```python
from build123d import *

# Parameters (mm, degrees)
F0_W          = 18
F0_H          = 32
F1_DEPTH      = 14
F2_W          = 13
F2_H          = 5
F2_W_2        = 2
F2_H_2        = 18.5
F3_DEPTH      = 14
F4_W          = 27
F4_H          = 6.5
F5_DEPTH      = 18.001
F6_R          = 1
F7_DEPTH      = 7.5
F8_R          = 1.25
F9_DEPTH      = 5
F10_T4_DEPTH  = 5
F11_T4_DEPTH  = 8.1066017178
F11_T9_DEPTH  = 8.1066017178
F11_T12_DEPTH = 20
F11_T14_DEPTH = 11.2132034356
F12_R         = 1
F13_T1_DEPTH  = 42.1410161514
F13_T3_DEPTH  = 42.5
F15_DEPTH     = 14.001
F16_R         = 1


# Not quite as in the source:
# - a fillet or chamfer that OpenCascade refuses, or shapes differently, is made with other operations: its cross-section is extruded or revolved along the edge and cut away or added


with BuildPart() as f1:
    # F0 (on Top) → F1 (new body)
    with BuildSketch(Plane.XY):
        with Locations((9, 16)):
            Rectangle(F0_W, F0_H)
    extrude(amount=F1_DEPTH)

    # F2 (on face) → F3 (cut, through all)
    with BuildSketch(Plane.XY.offset(14)):
        with Locations((11.5, 2.5)):
            Rectangle(F2_W, F2_H)
        with Locations((1, 22.75)):
            Rectangle(F2_W_2, F2_H_2)
    extrude(amount=-F3_DEPTH, mode=Mode.SUBTRACT)

    # F4 (on face) → F5 (cut, through all)
    with BuildSketch(Plane.YZ.offset(18)):
        with Locations((18.5, 3.25)):
            Rectangle(F4_W, F4_H)
    extrude(amount=-F5_DEPTH, mode=Mode.SUBTRACT)

    # F6 (on face) → F7 (cut, through all)
    with BuildSketch(Plane.XY.offset(14)):
        with Locations((13.5, 9.5)):
            Circle(F6_R)
        with BuildLine():
            ThreePointArc((18, 23.1904157598), (15.9251079936, 24.5306592691), (13.5, 25))
            ThreePointArc((13.5, 25), (7, 18.5), (13.5, 12))
            ThreePointArc((13.5, 12), (15.9251079936, 12.4693407309), (18, 13.8095842402))
            Line((18, 13.8095842402), (18, 23.1904157598))
        make_face()
        with Locations((13.5, 27.5)):
            Circle(F6_R)
        with BuildLine():
            Line((18, 25), (13.5, 25))
            ThreePointArc((13.5, 25), (15.9251079936, 24.5306592691), (18, 23.1904157598))
            Line((18, 23.1904157598), (18, 25))
        make_face()
        with BuildLine():
            ThreePointArc((18, 13.8095842402), (15.9251079936, 12.4693407309), (13.5, 12))
            Line((13.5, 12), (18, 12))
            Line((18, 12), (18, 13.8095842402))
        make_face()
    extrude(amount=-F7_DEPTH, mode=Mode.SUBTRACT)

    # F8 (on face) → F9 (cut, through all)
    with BuildSketch(Plane.YZ.offset(5)):
        with Locations((2.5, 11.55)):
            Circle(F8_R)
        with Locations((2.5, 2.95)):
            Circle(F8_R)
    extrude(amount=-F9_DEPTH, mode=Mode.SUBTRACT)

    # F10: chamfer of 8 on 1 edges, made by hand


with BuildPart() as f10_tool2:
    # F10_s3 → F10_t4 (new body)
    with BuildSketch(Plane.YZ.offset(5)):
        Polygon((5, -1.5), (13, 6.5), (5, 6.5), align=None)
    extrude(amount=-F10_T4_DEPTH)

    split(bisect_by=Plane.XY, keep=Keep.TOP)


with BuildPart() as f1_1:
    add(f1.part)

    # F10_t1: union F10_tool2
    add(f10_tool2.part)

    # F11: fillet of radius 3 on 5 edges, made by hand


with BuildPart() as f11_tool2:
    # F11_s3 → F11_t4 (new body)
    with BuildSketch(Plane.YZ.offset(5)):
        with BuildLine():
            ThreePointArc((14.2426406871, 6.5), (13.09459039, 6.2716385975), (12.1213203436, 5.6213203436))
            Line((12.1213203436, 5.6213203436), (13, 6.5))
            Line((13, 6.5), (14.2426406871, 6.5))
        make_face()
    extrude(amount=-F11_T4_DEPTH)

    split(bisect_by=Plane.YZ.offset(2), keep=Keep.TOP)


with BuildPart() as f1_2:
    add(f1_1.part)

    # F11_t1: union F11_tool2
    add(f11_tool2.part)


with BuildPart() as f11_tool7:
    # F11_s8 → F11_t9 (new body)
    with BuildSketch(Plane.YZ.offset(8.1066017178)):
        with BuildLine():
            ThreePointArc((14.2426406871, 6.5), (13.09459039, 6.2716385975), (12.1213203436, 5.6213203436))
            Line((12.1213203436, 5.6213203436), (13, 6.5))
            Line((13, 6.5), (14.2426406871, 6.5))
        make_face()
    extrude(amount=-F11_T9_DEPTH)

    split(bisect_by=Plane.YZ.offset(2), keep=Keep.BOTTOM)

    split(bisect_by=Plane.XZ.offset(-13.5), keep=Keep.TOP)


with BuildPart() as f1_3:
    add(f1_2.part)

    # F11_t6: union F11_tool7
    add(f11_tool7.part)

    # F11_s13 → F11_t12 (cut)
    with BuildSketch(Plane.YZ.offset(-7.5)):
        with BuildLine():
            ThreePointArc((0, 11), (0.8786796564, 13.1213203436), (3, 14))
            Line((3, 14), (0, 14))
            Line((0, 14), (0, 11))
        make_face()
        with BuildLine():
            ThreePointArc((0, 3), (0.8786796564, 0.8786796564), (3, 0))
            Line((3, 0), (0, 0))
            Line((0, 0), (0, 3))
        make_face()
    extrude(amount=F11_T12_DEPTH, mode=Mode.SUBTRACT)

    # F11_s15 → F11_t14 (cut)
    with BuildSketch(Plane.YZ.offset(-3.1066017178)):
        with BuildLine():
            ThreePointArc((7.3786796564, 0.8786796564), (6.40540961, 0.2283614025), (5.2573593129, 0))
            Line((5.2573593129, 0), (6.5, 0))
            Line((6.5, 0), (7.3786796564, 0.8786796564))
        make_face()
    extrude(amount=F11_T14_DEPTH, mode=Mode.SUBTRACT)

    # F12
    f12_edges = [f1_3.edges().sort_by_distance(p)[0] for p in [
        (18, 12, 10.25),
        (18, 25, 10.25),
    ]]
    fillet(f12_edges, radius=F12_R)

    # F13: fillet of radius 7 on 3 edges, made by hand

    # F13_s2 → F13_t1 (cut)
    with BuildSketch(Plane.XY.offset(-10.8205080757)):
        with BuildLine():
            ThreePointArc((18, 11), (15.6543724647, 6.7084973779), (11.0717967697, 5))
            Line((11.0717967697, 5), (11.0717967697, 4.86))
            Line((11.0717967697, 4.86), (18, 4.86))
            Line((18, 4.86), (18.14, 5))
            ThreePointArc((18.14, 5), (18.14, 8), (18.1385640646, 10.98))
            Line((18.1385640646, 10.98), (18, 11))
        make_face()
        with BuildLine():
            ThreePointArc((18, 26), (15.6543724647, 30.2915026221), (11.0717967697, 32))
            Line((11.0717967697, 32), (11.0717967697, 32.14))
            Line((11.0717967697, 32.14), (18, 32.14))
            Line((18, 32.14), (18.14, 32))
            ThreePointArc((18.14, 32), (18.14, 29), (18.1385640646, 26.02))
            Line((18.1385640646, 26.02), (18, 26))
        make_face()
    extrude(amount=F13_T1_DEPTH, mode=Mode.SUBTRACT)

    # F13_s4 → F13_t3 (cut)
    with BuildSketch(Plane.XY.offset(-11)):
        with BuildLine():
            ThreePointArc((9, 32), (4.0502525317, 29.9497474683), (2, 25))
            Line((2, 25), (1.86, 25))
            Line((1.86, 25), (1.86, 32.14))
            Line((1.86, 32.14), (9, 32.14))
            Line((9, 32.14), (9, 32))
        make_face()
    extrude(amount=F13_T3_DEPTH, mode=Mode.SUBTRACT)

    # F14 (on face) → F15 (cut, through all)
    with BuildSketch(Plane.XY.offset(14)):
        with BuildLine():
            ThreePointArc((8.1908098546, 14.75), (7, 18.5), (8.1908098546, 22.25))
            Line((8.1908098546, 22.25), (5.9908098546, 22.25))
            Line((5.9908098546, 22.25), (5.9908098546, 14.75))
            Line((5.9908098546, 14.75), (8.1908098546, 14.75))
        make_face()
    extrude(amount=-F15_DEPTH, mode=Mode.SUBTRACT)

    # F16
    f16_edges = [f1_3.edges().sort_by_distance(p)[0] for p in [
        (5.99081, 14.75, 10.25),
        (5.99081, 22.25, 10.25),
        (8.19081, 22.25, 10.25),
        (8.19081, 14.75, 10.25),
        (0, 13.5, 10.203314),
    ]]
    fillet(f16_edges, radius=F16_R)


solid = f1_3.part
```
Source: CAD feature listing. Evaluate the final solid. Frame: model axes, mm. A direction names the side the tool comes from. Give positions to 0.01 mm unless a question says otherwise; leave off trailing zeros. Write each loop counter-clockwise with the first axis right and the second up, starting at its lowest first coordinate (ties: lowest second). Pieces come first, ordered by that corner, then holes.
1. Section query C-C (x = 14). Return the cut outline in (y, z).
2. Section query B-B (y = 27.5). Return the cut outline in (x, z), then the cut area to 3 significant figures.
3. Section query D-D (x = 11.75). Return the cut outline in (y, z).
4. Pull-direction query (Y, two-part tool) for faces 1 (the face through (2.535, 3.077, 1.841)), 2 (the face through (5, 18, 14)), 3 (the face through (8, 5, 10)), 4 (the face through (10.681, 12.643, 10.302)); classes: +Y half, -Y half, draft (parallel to the pull), parting line (faces both ways), or undercut.
5. First-contact query: pin 1 (1.8 mm diameter, centred on x = 15.5, z = 9.5, fed in from -Y); pin 2 (5 mm diameter, centred on x = 9, z = 10.5, fed in from -Y); pin 3 (6 mm diameter, centred on y = 19.5, z = 11, fed in from -X). Flat tips, straight axial feed; report the tip coordinate or a pass-through.
6. Section query A-A (z = 11.55). Count the separate pieces of the cut face and the enclosed holes in it, then the cut area to 3 significant figures.
7. Material intervals for line 1 along Y through (x, z) = (13.5, 10.5); line 2 along Z through (x, y) = (3.7, 2.5); line 3 along X through (y, z) = (21, 8.5), sorted ascending.
8. Access query for faces 5 (the face through (17.715, 25.301, 10.198)), 6 (the face through (5, 18, 6.5)), 7 (the face through (3.091, 12.872, 6.169)), 8 (the face through (2, 19, 10)). Directions: +Z, -Z, +X, -X, +Y, -Y. A direction counts if a zero-diameter tool reaches every point of the face in a straight line with its end or side. Return the directions, or none.
Output values:
1. outline: (5.64, 6.5) - (8.63, 6.5) - (8.63, 14) - (5.64, 14) - close; (10.37, 6.5) - (12, 6.5) - (12, 14) - (10.37, 14) - close; (25, 6.5) - (26.63, 6.5) - (26.63, 14) - (25, 14) - close; (28.37, 6.5) - (31.36, 6.5) - (31.36, 14) - (28.37, 14) - close
2. outline: (2.46, 6.5) - (12.5, 6.5) - (12.5, 14) - (2.46, 14) - close; (14.5, 6.5) - (17.61, 6.5) - (17.61, 14) - (14.5, 14) - close
2. area: 98.6 mm2
3. outline: (5.03, 6.5) - (12.24, 6.5) - (12.24, 14) - (5.03, 14) - close; (24.76, 6.5) - (31.97, 6.5) - (31.97, 14) - (24.76, 14) - close
4. face 1: undercut
4. face 2: draft
4. face 3: -Y half
4. face 4: undercut
5. pin 1: stops at y = 5.95
5. pin 2: stops at y = 5
5. pin 3: stops at x = 2
6. separate pieces: 2
6. enclosed holes: 2
6. area: 289 mm2
7. line 1: y = 5.43 to 8.5, 10.5 to 12, 25 to 26.5, 28.5 to 31.57
7. line 2: z = 0.04 to 1.7, 4.2 to 10.3, 12.8 to 13.96
7. line 3: x = 2 to 5.99
8. face 5: +Z, -Z, +X
8. face 6: -Z, +X, +Y
8. face 7: -Z, +X, -X, +Y
8. face 8: +Z, -Z, -X, +Y
